Geometry check sheet. Reference: drawing and pictorial views, mm from the part's lowest x, y, z. Round coordinates to 2 decimals unless told otherwise and drop trailing zeros. Order: outer loops, then holes, each group sorted by start corner. A loop starts at its lowest first (then second) coordinate and runs counter-clockwise, first axis right, second up.
(1) Thickness scan on probe 1 along X at (y, z) = (1.2, 43.5); probe 2 along Z at (x, y) = (3.5, 1.3); probe 3 along X at (y, z) = (1.35, 12). Record the ranges inside material, lowest first.
(2) Sectioned sample at B-B, the plane x = 56. Enter the section's corners in (y, z), and give its area (3 significant figures).
(3) Depth check by flat-ended pin: pin 1 (0.6 mm diameter, centred on y = 0.5, z = 1.5, fed in from -X); pin 2 (1 mm diameter, centred on x = 40, y = 1.5, fed in from +Z); pin 3 (1 mm diameter, centred on y = 1.5, z = 2, fed in from +X). Enter the tip coordinate at first touch or a pass-through.
(4) Sectioned sample at A-A, the plane z = 35. Enter the section's corners in (x, y), and give its area (3 significant figures).
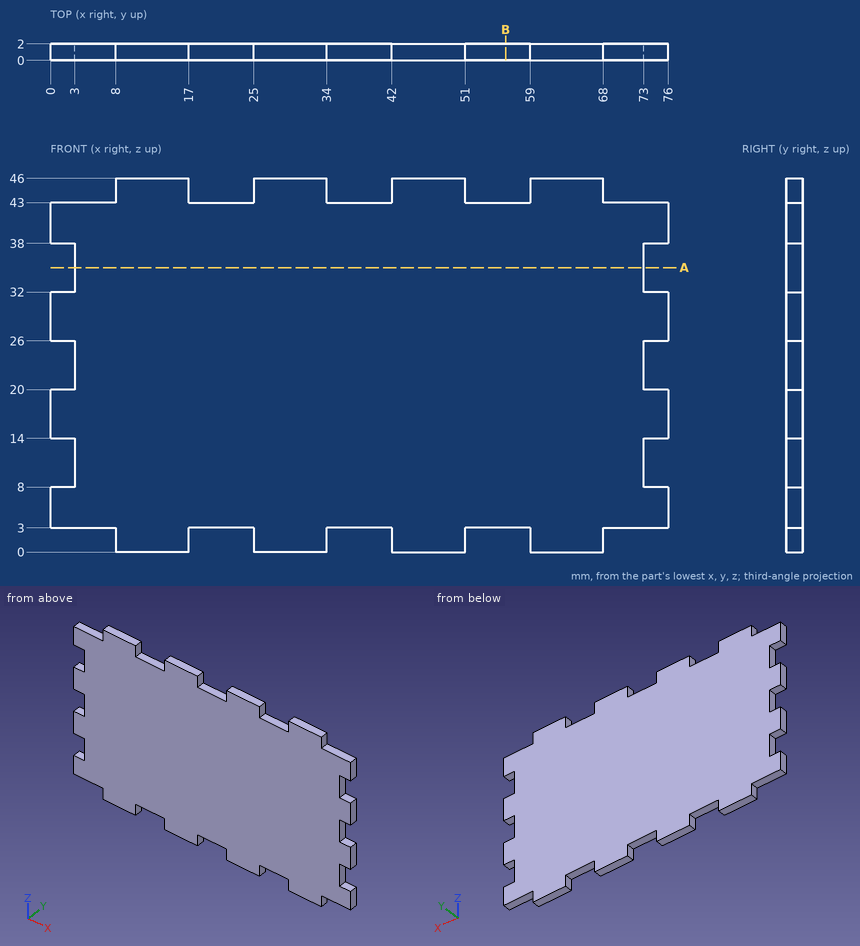
Derived:
1. probe 1: x = 8 to 17, 25 to 34, 42 to 51, 59 to 68
1. probe 2: z = 3 to 43
1. probe 3: x = 3 to 73
2. outline: (0, 3) - (2, 3) - (2, 43) - (0, 43) - close
2. area: 80.0 mm2
3. pin 1: stops at x = 8
3. pin 2: stops at z = 43
3. pin 3: stops at x = 68
4. outline: (3, 0) - (73, 0) - (73, 2) - (3, 2) - close
4. area: 140 mm2
